Model file for the job. Use its own axes, mm. A direction names the side the tool comes from. Round coordinates to 2 decimals unless told otherwise and drop trailing zeros. Loops run counter-clockwise (first coordinate to the right, second up) from the corner with the lowest first, then second, coordinate; pieces in that order, holes last. Notation, with made-up numbers: M 27,19.25 L 60,19.25 A33 cw 60,48.25 Z; hole C 68.5,-3.5 d7. An arc over 180 degrees is marked long. Answer in a Markdown table with one row per item.
from build123d import *

# Parameters (mm, degrees)
F1_DEPTH = 53.975
F3_DEPTH = 25.4
F4_W     = 16.1045007408
F4_H     = 10.7811614871
F5_DEPTH = 3.175
F6_W     = 3.2399867196
F6_H     = 27.9691088945
F7_REACH = 124.3150351858
F8_W     = 26.4270068914
F8_H     = 19.5576284379
F9_DEPTH = 3.175
F10_R    = 5.08
F11_R    = 2.54


with BuildPart() as f1:
    # F0 (on Right) → F1 (new body)
    with BuildSketch(Plane.YZ):
        with BuildLine():
            Line((0, 0), (56.8904802203, 0))
            Line((56.8904802203, 0), (56.8904802203, 3.175))
            Line((56.8904802203, 3.175), (14.4803198381, 3.175))
            ThreePointArc((14.4803198381, 3.175), (8.981058524, 6.35), (8.981058524, 12.7))
            Line((8.981058524, 12.7), (56.5364878665, 95.0684197969))
            Line((56.5364878665, 95.0684197969), (53.4993190127, 96.1578890309))
            Line((53.4993190127, 96.1578890309), (0, 3.4943503306))
            Line((0, 3.4943503306), (0, 0))
        make_face()
    extrude(amount=F1_DEPTH)

    # F2 (on face) → F3 (join)
    with BuildSketch(Plane(origin=(0, -1.513098078, 0.8735875827), x_dir=(1, 0, 0), z_dir=(0, -0.8660254038, 0.5))):
        Polygon((27.5479931086, 17.2171894163), (53.975, 17.2171894163), (53.975, 36.7748178542), (50.8, 36.7748178542), (50.8, 20.3921894163), (27.5479931086, 20.3921894163), align=None)
    extrude(amount=F3_DEPTH)

    # F4 (on face) → F5 (cut, through all)
    with BuildSketch(Plane(origin=(0, -1.513098078, 0.8735875827), x_dir=(1, 0, 0), z_dir=(0, -0.8660254038, 0.5))):
        with Locations((8.0522503704, 38.3052378893)):
            Rectangle(F4_W, F4_H)
    extrude(amount=-F5_DEPTH, mode=Mode.SUBTRACT)

    f7_end = Plane(origin=(8.0522503704, 16.3190458234, 28.5847668277), x_dir=(0, 0.8660254038, -0.5), z_dir=(0, 0.5, 0.8660254038))
    # F6 (on Top) → F7 (cut, up to a plane its end follows)
    with BuildSketch(Plane.XY):
        with Locations((1.6199933598, 13.9845544472)):
            Rectangle(F6_W, F6_H)
    f7_long = extrude(amount=F7_REACH, mode=Mode.PRIVATE)
    add(split(f7_long, bisect_by=f7_end, keep=Keep.BOTTOM, mode=Mode.PRIVATE), mode=Mode.SUBTRACT)

    # F8 (on face) → F9 (join)
    with BuildSketch(Plane(origin=(0, -23.5101433341, 13.5735875827), x_dir=(1, 0, 0), z_dir=(0, -0.8660254038, 0.5))):
        with Locations((40.7614965543, 26.9960036352)):
            Rectangle(F8_W, F8_H)
    extrude(amount=F9_DEPTH)

    # F10
    f10_edges = [f1.edges().sort_by_distance(p)[0] for p in [
        (28.607493, 0, 3.49435),
        (53.975, -5.277841, 22.927861),
        (27.547993, -6.49755, 46.215264),
    ]]
    fillet(f10_edges, radius=F10_R)

    # F11
    f11_edges = [f1.edges().sort_by_distance(p)[0] for p in [
        (53.975, 55.017903, 95.613154),
        (53.975, 56.89048, 1.5875),
        (3.239987, 16.319046, 28.584767),
    ]]
    fillet(f11_edges, radius=F11_R)

    # F12: F1 across plane


with BuildPart() as f1_1:
    add(f1.part)
    add(f1.part.mirror(Plane.YZ))


solid = f1_1.part
1. Saw through at B-B (z = 9). Write the cut outline in (x, y) (3 decimals), and give its area (3 significant figures).
Verdict:
| item | result |
|---|---|
| outline | M -53.975,3.179 L -3.24,3.179 L -3.24,8.152 L -53.975,8.152 Z; M 3.24,3.179 L 53.975,3.179 L 53.975,8.152 L 3.24,8.152 Z |
| area | 505 mm² |
2. Pin check, flat tips, straight feed: pin 1 (1.1 mm diameter, centred on x = 16, z = 1.5, fed in from -Y); pin 2 (10 mm diameter, centred on x = -21.5, z = 57, fed in from +Y); pin 3 (8 mm diameter, centred on x = -14, z = 84, fed in from +Y). Stop position of each tip, or through.
Verdict:
| item | result |
|---|---|
| pin 1 | stops at y = 0 |
| pin 2 | stops at y = 37.44 |
| pin 3 | stops at y = 52.46 |
3. Tool access for faces 1 (the flat face through (-27.548, -7, 27)), 2 (the flat face through (1, 36, 3.175)), 3 (the flat face through (-39.01, -9.16, 38.43)), 4 (the cylindrical face through (-28.96, 0.18, 3.47)): list every direction of +Z, -Z, +X, -X, +Y, -Y with a clear straight run to the whole face (end or side of a thin tool).
Verdict:
| item | result |
|---|---|
| face 1 | +Z, -Y |
| face 2 | +X, -X, +Y |
| face 3 | none |
| face 4 | +X, -X, -Y |
4. Mould opens along Z. For faces 5 (the cylindrical face through (4.004, 15.976, 27.946)), 6 (the flat face through (-3.24, 9, 6)), 7 (the flat face through (39.337, -2.162, 24.795)) say: +Z half, -Z half, draft (parallel to the pull), parting line (faces both ways), or undercut.
Verdict:
| item | result |
|---|---|
| face 5 | +Z half |
| face 6 | draft |
| face 7 | undercut |
5. Saw through at C-C (x = -25.5). Write the cut outline in (y, z) (3 decimals), and give its area (3 significant figures).
Verdict:
| item | result |
|---|---|
| outline | M 0,0 L 56.89,0 L 56.89,3.175 L 14.48,3.175 A6.35 cw 8.981,12.7 L 56.536,95.068 L 53.499,96.158 L 0.681,4.673 A5.08 ccw 0,2.133 Z |
| area | 547 mm² |
6. Saw through at A-A (x = 0). Write the cut outline in (y, z) (3 decimals).
Verdict:
| item | result |
|---|---|
| outline | M 20.335,38.715 L 23.084,37.128 L 56.536,95.068 L 53.499,96.158 Z; M 27.969,0 L 56.89,0 L 56.89,3.175 L 27.969,3.175 Z |
7. Wall check: probe 1 along X at (y, z) = (-9, 34) (3 decimals); probe 2 along Z at (x, y) = (-7, 33) (3 decimals); probe 3 along Z at (x, y) = (13, 42.5) (1 decimal). Give the ranges that are in metal, low to high.
Verdict:
| item | result |
|---|---|
| probe 1 | x = -53.975 to -50.8, 50.8 to 53.975 |
| probe 2 | z = 0 to 3.175, 54.302 to 60.652 |
| probe 3 | z = 0 to 3.2, 70.8 to 77.1 |
